The listing builds one solid part. Answer for the finished solid, in the listing's coordinates (mm). Face numbers are marked on the shaded views. A direction names the side the tool comes from. Give positions to 0.01 mm unless a question says otherwise; leave off trailing zeros. Loops run counter-clockwise (first coordinate to the right, second up) from the corner with the lowest first, then second, coordinate; pieces in that order, holes last.
Item 1: Consider line 1 along Y through (x, z) = (2, 0.5); line 2 along Z through (x, y) = (-1.25, -21); line 3 along Z through (x, y) = (-0.5, -30.5). Determine where each line is inside the solid, lowest interval first.
Item 2: A tool of negligible diameter and unlimited length cuts with its end or side. For the marked faces 1 and 2, from which of +Z, -Z, +X, -X, +Y, -Y can it reach the whole face along a straight path? Write none if from no direction.
Item 3: Section A-A, the plane z = -0.5 is taken. Give the vertices of the cut face in (x, y), and give its area (3 significant figures).
Item 4: Each of these flat-tipped pins is pushed along its axis until it touches: pin 1 Ø1 at (x, y) = (-0.5, -28.5) entering from -Z; pin 2 Ø3.5 at (x, z) = (-1, -0.5) entering from +Y; pin 3 Ø1 at (x, y) = (1.5, -10.5) entering from -Z; pin 4 Ø1 at (y, z) = (-28.5, 0) entering from +X. Where does it stop, or does it pass through?
Item 5: Section B-B, the plane y = -30 is taken. Give the vertices of the cut face in (x, z).
Item 6: Section C-C, the plane z = 3 is taken. Give the vertices of the cut face in (x, y).
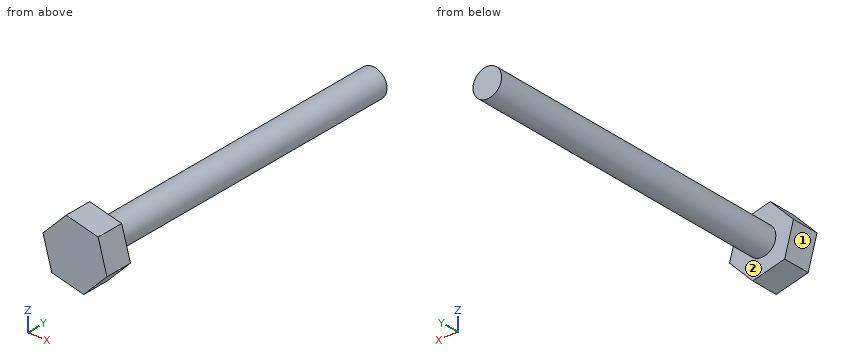
from build123d import *

# Parameters (mm, degrees)
BOSS_EXTRU_1_DEPTH = 3
ESQUISSE2_W        = 1.5
ESQUISSE2_H        = 35


with BuildPart() as part:
    # Esquisse1 → Boss.-Extru.1 (new body)
    with BuildSketch(Plane.XZ.offset(38)):
        Polygon((0.924188604, -3.338543908), (3.353358138, -0.868901145), (2.429169534, 2.469642763), (-0.924188604, 3.338543908), (-3.353358138, 0.868901145), (-2.429169534, -2.469642763), align=None)
    extrude(amount=-BOSS_EXTRU_1_DEPTH)

    # Esquisse2 → Révolution1 (revolve)
    with BuildSketch(Plane(origin=(0, 0, 0), x_dir=(-1, 0, 0), z_dir=(0, 0, -1)), mode=Mode.PRIVATE) as r_volution1_sk:
        with Locations((-0.75, -17.5)):
            Rectangle(ESQUISSE2_W, ESQUISSE2_H)
    revolve(r_volution1_sk.sketch.rotate(Axis((0, -35, 0), (0, 1, 0)), 270), axis=Axis((0, -35, 0), (0, 1, 0)))


solid = part.part
Worked answers:
1. line 1: y = -38 to -35
1. line 2: z = -0.83 to 0.83
1. line 3: z = -1.41 to 1.41
2. face 1: -Z, -X, +Y, -Y
2. face 2: +Y
3. outline: (-2.97, -38) - (3.25, -38) - (3.25, -35) - (1.41, -35) - (1.41, 0) - (-1.41, 0) - (-1.41, -35) - (-2.97, -35) - close
3. area: 118 mm2
4. pin 1: stops at z = -1.5
4. pin 2: stops at y = 0
4. pin 3: stops at z = -1.12
4. pin 4: stops at x = 1.5
5. outline: circle Ø3 at (0, 0)
6. outline: (-1.26, -38) - (0.38, -38) - (0.38, -35) - (-1.26, -35) - close
